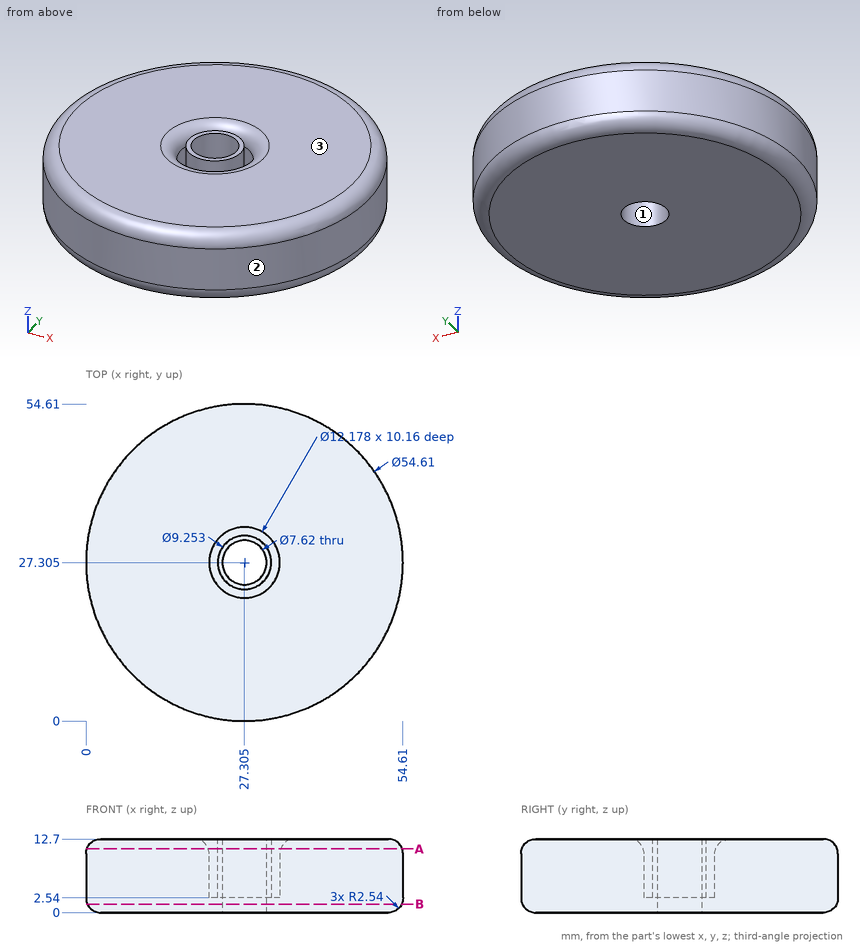
Input: dimensioned drawing with shaded views. Units: mm. Origin: part minimum x, y, z. Coordinates: 2 decimals unless noted, no trailing zeros. Order: outer loops, then holes, each group sorted by start corner. A loop starts at its lowest first (then second) coordinate and runs counter-clockwise, first axis right, second up. Notation, with made-up numbers: (-5.75, 75) - (5.25, 75) arc R27 cw to (5.25, 93) - close; hole circle Ø3 at (43.25, 55). An arc over 180 degrees is marked (long way). Put each result on its own line as item: value.
1. Contact query for flat-ended pins moving along their axis: pin 1 Ø1 at (x, z) = (23.5, 11) entering from -Y (1 decimal); pin 2 Ø4.5 at (x, y) = (27.305, 27.305) entering from +Z; pin 3 Ø3 at (x, z) = (22.5, 5) entering from +Y; pin 4 Ø6 at (y, z) = (41.5, 9) entering from +X. Output: stop coordinate, or through.
Report:
pin 1: stops at y = 0.3
pin 2: passes through
pin 3: stops at y = 54.41
pin 4: stops at x = 52.21
2. Draft query along X for the marked faces 1, 2 and 3. Return one class per face: pulls with the +X half, pulls with the -X half, needs draft (parallel to the pull), parting line crosses it, or undercut.
Report:
face 1: undercut
face 2: parting line crosses it
face 3: needs draft
3. Cut plane A-A on z = 11. Return the cut outline in (x, y) (1 decimal), then the cut area to 3 significant figures.
Report:
outline: circle Ø54.3 at (27.3, 27.3); circle Ø9.3 at (27.3, 27.3); hole circle Ø12.5 at (27.3, 27.3); hole circle Ø7.6 at (27.3, 27.3)
area: 2,220 mm2
4. Cut plane B-B on z = 1.5. Return the cut outline in (x, y) (1 decimal), then the cut area to 3 significant figures.
Report:
outline: circle Ø54.2 at (27.3, 27.3); hole circle Ø7.6 at (27.3, 27.3)
area: 2,260 mm2
5. Line query: line 1 along X through (y, z) = (27, 5); line 2 along X through (y, z) = (29, 6.25) (1 decimal); line 3 along Y through (x, z) = (22, 4.75) (1 decimal). Output: solid intervals per line, ascending.
Report:
line 1: x = 0 to 21.22, 22.69 to 23.51, 31.1 to 31.92, 33.39 to 54.61
line 2: x = 0.1 to 21.5, 23 to 23.9, 30.7 to 31.6, 33.2 to 54.6
line 3: y = 0.5 to 24.3, 30.3 to 54.1
